from build123d import *

# Parameters (mm, degrees)
F0_W     = 180
F0_H     = 100
F1_DEPTH = 10
F2_R     = 5
F3_W     = 30
F3_H     = 30
F4_DEPTH = 10
F5_R     = 5
F6_DEPTH = 5


with BuildPart() as f1:
    # F0 (on Front) → F1 (new body)
    with BuildSketch(Plane.XZ):
        Rectangle(F0_W, F0_H)
    extrude(amount=F1_DEPTH)

    # F2
    f2_edges = [f1.edges().sort_by_distance(p)[0] for p in [
        (0, -10, 50),
        (-90, -10, 0),
        (0, -10, -50),
        (90, -10, 0),
    ]]
    fillet(f2_edges, radius=F2_R)

    # F3 (on face) → F4 (join)
    with BuildSketch(Plane.XZ.offset(10)):
        Rectangle(F3_W, F3_H)
    extrude(amount=F4_DEPTH)

    # F5 (on face) → F6 (join)
    with BuildSketch(Plane.XZ.offset(20)):
        Circle(F5_R)
    extrude(amount=F6_DEPTH)


solid = f1.part
Work out the finished part from the listing and answer in its coordinate system (mm). A direction names the side the tool comes from. Give positions to 0.01 mm unless a question says otherwise; leave off trailing zeros. Loops run counter-clockwise (first coordinate to the right, second up) from the corner with the lowest first, then second, coordinate; pieces in that order, holes last. Notation, with made-up numbers: (79, 40) -> (100, 40) arc R36 cw to (100, 79) -> close; hole circle Ø7 at (15.25, -34.5). An arc over 180 degrees is marked (long way). Use a Markdown table: item, result. Add a question column.
1. Section C-C on y = -18 is taken. Determine the outline of the cut face in (x, z).
2. Section B-B on z = 0 is taken. Determine the outline of the cut face in (x, y).
3. Find the intervals of material crossed by probe 1 along Z at (x, y) = (8.5, -18.75); probe 2 along Y at (x, z) = (27.5, 45.5); probe 3 along Y at (x, z) = (-8, 10), in increasing order.
4. Flat-ended cylindrical pins translate along their axes: pin 1 Ø8 at (x, z) = (16, -3) entering from -Y; pin 2 Ø3 at (x, y) = (-1, -16.5) entering from -Z; pin 3 Ø5 at (x, y) = (-0.5, -13.5) entering from +Z; pin 4 Ø1.5 at (x, z) = (-27.5, 22) entering from +Y. Find the tip coordinate at first contact, or state that the pin passes through.
5. For faces 1 (the flat face through (0, -15, -15)), 2 (the flat face through (15, -15, 0)), 3 (the flat face through (-15, -15, 0)), 4 (the cylindrical face through (-1.08, -22.46, -4.88)), determine the directions among +Z, -Z, +X, -X, +Y, -Y from which every point of the face is accessible in a straight line to the end or side of a thin tool.
6. Section A-A on x = 0 is taken. Determine the outline of the cut face in (y, z).
7. Section D-D on x = -20 is taken. Determine the outline of the cut face in (y, z), and give its area (3 significant figures).
Results below:
| question | item | result |
|---|---|---|
| 1 | outline | (-15, -15) -> (15, -15) -> (15, 15) -> (-15, 15) -> close |
| 2 | outline | (-90, -5) arc R5 ccw to (-85, -10) -> (-15, -10) -> (-15, -20) -> (-5, -20) -> (-5, -25) -> (5, -25) -> (5, -20) -> (15, -20) -> (15, -10) -> (85, -10) arc R5 ccw to (90, -5) -> (90, 0) -> (-90, 0) -> close |
| 3 | probe 1 | z = -15 to 15 |
| 3 | probe 2 | y = -9.97 to 0 |
| 3 | probe 3 | y = -20 to 0 |
| 4 | pin 1 | stops at y = -20 |
| 4 | pin 2 | stops at z = -15 |
| 4 | pin 3 | stops at z = 15 |
| 4 | pin 4 | stops at y = 0 |
| 5 | face 1 | -Z, +X, -X, -Y |
| 5 | face 2 | +Z, -Z, +X, -Y |
| 5 | face 3 | +Z, -Z, -X, -Y |
| 5 | face 4 | -Y |
| 6 | outline | (-25, -5) -> (-20, -5) -> (-20, -15) -> (-10, -15) -> (-10, -45) arc R5 ccw to (-5, -50) -> (0, -50) -> (0, 50) -> (-5, 50) arc R5 ccw to (-10, 45) -> (-10, 15) -> (-20, 15) -> (-20, 5) -> (-25, 5) -> close |
| 7 | outline | (-10, -45) arc R5 ccw to (-5, -50) -> (0, -50) -> (0, 50) -> (-5, 50) arc R5 ccw to (-10, 45) -> close |
| 7 | area | 989 mm^2 |
